```python
from build123d import *

# Parameters (mm, degrees)
F1_DEPTH = 2.286
F2_DEPTH = 8.636
F3_W     = 67.638885
F3_H     = 6.652117
F4_DEPTH = 57.658
F5_R     = 3.239595
F6_DEPTH = 25.4


with BuildPart() as f1:
    # F0 (on Front) → F1 (new body)
    with BuildSketch(Plane.XZ):
        Polygon((35.56, 35.56), (0, 35.56), (-35.56, 35.56), (-35.56, -22.86), (35.56, -22.86), align=None)
    extrude(amount=F1_DEPTH)

    # F0 (on Front) → F2 (join)
    with BuildSketch(Plane.XZ):
        Polygon((35.56, 35.56), (0, 35.56), (-35.56, 35.56), (-35.56, -22.86), (35.56, -22.86), align=None)
    extrude(amount=-F2_DEPTH)

    # F3 (on face) → F4 (cut)
    with BuildSketch(Plane(origin=(0, 0, -22.86), x_dir=(1, 0, 0), z_dir=(0, 0, -1))):
        with Locations((0.041259, -3.326058)):
            Rectangle(F3_W, F3_H)
    extrude(amount=-F4_DEPTH, mode=Mode.SUBTRACT)

    # F5 (on face) → F6 (cut)
    with BuildSketch(Plane.XZ.offset(2.286)):
        Circle(F5_R)
    extrude(amount=-F6_DEPTH, mode=Mode.SUBTRACT)


solid = f1.part
```
For this review, take the finished solid that the model builds, in its own axes (mm). A direction names the side the tool comes from. Coordinates: 2 decimals unless noted, no trailing zeros. Loops run counter-clockwise (first coordinate to the right, second up) from the corner with the lowest first, then second, coordinate; pieces in that order, holes last. Notation, with made-up numbers: (22, 27.5) - (79, 27.5) arc R28 cw to (79, 54.5) - close; hole circle Ø1 at (73.25, -1.5). An arc over 180 degrees is marked (long way). Use one line per item in the form item = value. Start each with the question number.
1) For faces 1 (the face through (0, 8.636, 7)), 2 (the face through (-33.778, 3, 6)), list the 3-axis set-ups (+Z, -Z, +X, -X, +Y, -Y) from which the entire face can be reached by the end or side of a thin tool; tool diameter is ignored.
2) Take a section at D-D (y = 4.75). State the section outline as (x, z) points, plus the area to 3 significant figures.
3) Draft analysis for pull direction Z (two halves, no side actions). For faces 3 (the face through (0, 3, 34.798)), 4 (the face through (-0.702, -1.159, -3.163)), 5 (the face through (0, 3, 35.56)), 6 (the face through (33.861, 3, 6)), state which applies: released by +Z, released by -Z, zero draft, split by the parting line, or undercut.
4) Take a section at C-C (z = -11.5). State the section outline as (x, y) points.
5) To check wall thickness, follow probe 1 along X at (y, z) = (4.5, -18.5); probe 2 along Z at (x, y) = (0, 7.65); probe 3 along Y at (x, z) = (-5.5, 22.5). State the ranges of each line that lie inside material, in increasing order. Write a range as from..to.
6) Take a section at B-B (x = 0). State the section outline as (y, z) points, plus the area to 3 significant figures.
7) Take a section at A-A (z = 0). State the section outline as (x, y) points.
From the geometry:
q1.face_1 = +Z, -Z, +X, -X, +Y
q1.face_2 = -Z
q2.outline = (-35.56, -22.86) - (-33.78, -22.86) - (-33.78, 34.8) - (33.86, 34.8) - (33.86, -22.86) - (35.56, -22.86) - (35.56, 35.56) - (-35.56, 35.56) - close
q2.area = 255 mm2
q3.face_3 = released by -Z
q3.face_4 = undercut
q3.face_5 = released by +Z
q3.face_6 = zero draft
q4.outline = (-35.56, -2.29) - (35.56, -2.29) - (35.56, 8.64) - (-35.56, 8.64) - close; hole (-33.78, 0) - (33.86, 0) - (33.86, 6.65) - (-33.78, 6.65) - close
q5.probe_1 = -35.56..-33.78, 33.86..35.56
q5.probe_2 = -22.86..-3.24, 3.24..35.56
q5.probe_3 = -2.29..0, 6.65..8.64
q6.outline = (-2.29, -22.86) - (0, -22.86) - (0, -3.24) - (-2.29, -3.24) - close; (-2.29, 3.24) - (0, 3.24) - (0, 34.8) - (6.65, 34.8) - (6.65, 3.24) - (8.64, 3.24) - (8.64, 35.56) - (-2.29, 35.56) - close; (6.65, -22.86) - (8.64, -22.86) - (8.64, -3.24) - (6.65, -3.24) - close
q6.area = 227 mm2
q7.outline = (-35.56, -2.29) - (-3.24, -2.29) - (-3.24, 0) - (-33.78, 0) - (-33.78, 6.65) - (-3.24, 6.65) - (-3.24, 8.64) - (-35.56, 8.64) - close; (3.24, -2.29) - (35.56, -2.29) - (35.56, 8.64) - (3.24, 8.64) - (3.24, 6.65) - (33.86, 6.65) - (33.86, 0) - (3.24, 0) - close
